Source: CAD feature listing. Evaluate the final solid. Frame: model axes, mm. A direction names the side the tool comes from. Round coordinates to 2 decimals unless told otherwise and drop trailing zeros. Loops run counter-clockwise (first coordinate to the right, second up) from the corner with the lowest first, then second, coordinate; pieces in that order, holes last. Notation, with made-up numbers: (-29, 32.25) - (-21, 32.25) arc R35 cw to (-21, 68.25) - close; hole circle Ø5 at (73, 66.25). An arc over 180 degrees is marked (long way). One line per question, with ' | ' between items. Start each with the question number.
1. Access query for faces 5 (the flat face through (-10, 7, 2)), 6 (the flat face through (-20, 70, 5)), 7 (the flat face through (13, 20, 5)). Directions: +Z, -Z, +X, -X, +Y, -Y. A direction counts if a zero-diameter tool reaches every point of the face in a straight line with its end or side. Return the directions, or none.
2. Cut plane D-D (z = 1). Return loops of the section in (x, y), then the cut area to 3 significant figures.
3. Cut plane C-C (z = -10). Return loops of the section in (x, y), then the cut area to 3 significant figures.
4. Pin query (flat end, axial travel): pin 1 (10 mm diameter, centred on y = 10.5, z = 4.5, fed in from +X); pin 2 (6.5 mm diameter, centred on x = 1, y = 43.5, fed in from +Z); pin 3 (3 mm diameter, centred on x = 14.5, y = 42, fed in from -Z); pin 4 (5 mm diameter, centred on x = 0, y = 47.5, fed in from -Z). Return the tip coordinate at first contact, or that it passes through.
5. Mould query, pull axis Y, two halves, no side actions, for faces 1 (the flat face through (0, 4, -13)), 2 (the flat face through (25, 47, 5)), 3 (the cylindrical face through (-2.379, 36.786, 6.549)), 4 (the cylindrical face through (0.14, 0.57, 9.4)). Classes: pulls with the +Y half, pulls with the -Y half, needs draft (parallel to the pull), parting line crosses it, or undercut.
6. Cut plane B-B (x = 0). Return loops of the section in (y, z) (3 decimals), then the cut area to 3 significant figures.
7. Cut plane A-A (y = 47.5). Return loops of the section in (x, z) (3 decimals).
8. Ray query, line 1 (Y direction, x = 0, z = 1.1); line 2 (Y direction, x = 0, z = 5.75) (3 decimals); line 3 (X direction, y = 1.1, z = -10). Return the intervals inside material, ascending.
```python
from build123d import *

# Parameters (mm, degrees)
SCHIZZO1_R                   = 4
ESTRUSIONE_ESTRUSIONE1_DEPTH = 10
SMUSSO1_SIZE                 = 10
SCHIZZO3_R                   = 10.975
TAGLIO_ESTRUSIONE1_DEPTH     = 7
SCHIZZO4_W                   = 20
SCHIZZO4_H                   = 4
ESTRUSIONE_ESTRUSIONE2_DEPTH = 20
RACCORDO1_R                  = 2
SCHIZZO5_R                   = 2.5
TAGLIO_ESTRUSIONE2_DEPTH     = 20
SCHIZZO6_R                   = 2.5
TAGLIO_ESTRUSIONE3_DEPTH     = 11


with BuildPart() as part:
    # Schizzo1 → Estrusione-Estrusione1 (new body)
    with BuildSketch(Plane.XY):
        Polygon((-25, 20), (-10, 20), (-10, 0), (10, 0), (10, 20), (25, 20), (25, 75), (-25, 75), align=None)
        with Locations((0, 47.5)):
            Circle(SCHIZZO1_R, mode=Mode.SUBTRACT)
    extrude(amount=ESTRUSIONE_ESTRUSIONE1_DEPTH)

    # Smusso1
    smusso1_edges = [part.edges().sort_by_distance(p)[0] for p in [
        (25, 20, 5),
        (-25, 20, 5),
        (-25, 75, 5),
        (25, 75, 5),
    ]]
    chamfer(smusso1_edges, length=SMUSSO1_SIZE)

    # Schizzo3 → Taglio-Estrusione1 (cut)
    with BuildSketch(Plane.XY.offset(10)):
        with Locations((0, 47.5)):
            Circle(SCHIZZO3_R)
    extrude(amount=-TAGLIO_ESTRUSIONE1_DEPTH, mode=Mode.SUBTRACT)

    # Schizzo4 → Estrusione-Estrusione2 (add)
    with BuildSketch(Plane(origin=(0, 0, 0), x_dir=(-1, 0, 0), z_dir=(0, 0, -1))):
        with Locations((0, 2)):
            Rectangle(SCHIZZO4_W, SCHIZZO4_H)
    extrude(amount=ESTRUSIONE_ESTRUSIONE2_DEPTH)

    # Raccordo1
    raccordo1_edges = [part.edges().sort_by_distance(p)[0] for p in [
        (10, 20, 5),
        (-10, 20, 5),
        (0, 0, 10),
        (0, 4, 0),
        (10, 2, -20),
        (-10, 2, -20),
    ]]
    fillet(raccordo1_edges, radius=RACCORDO1_R)

    # Schizzo5 → Taglio-Estrusione2 (cut)
    with BuildSketch(Plane(origin=(0, 4, 0), x_dir=(1, 0, 0), z_dir=(0, 1, 0))):
        with Locations((0, 10)):
            Circle(SCHIZZO5_R)
    extrude(amount=-TAGLIO_ESTRUSIONE2_DEPTH, mode=Mode.SUBTRACT)

    # Schizzo6 → Taglio-Estrusione3 (cut, through all)
    with BuildSketch(Plane(origin=(0, 0, 0), x_dir=(-1, 0, 0), z_dir=(0, 0, -1))):
        with Locations((0, 10)):
            Circle(SCHIZZO6_R)
    extrude(amount=-TAGLIO_ESTRUSIONE3_DEPTH, mode=Mode.SUBTRACT)


solid = part.part
```
Answers follow:
1) face 5: +Z, -Z, -X, -Y | face 6: +Z, -Z, -X, +Y | face 7: +Z, -Z, +X, -Y
2) outline: (-25, 30) - (-15, 20) - (-12, 20) arc R2 cw to (-10, 18) - (-10, 0) - (10, 0) - (10, 18) arc R2 cw to (12, 20) - (15, 20) - (25, 30) - (25, 65) - (15, 75) - (-15, 75) - (-25, 65) - close; hole circle Ø8 at (0, 47.5); hole circle Ø5 at (0, 10) | area: 2,880 mm2
3) outline: (-10, 0) - (-2.5, 0) - (-2.5, 4) - (-10, 4) - close; (2.5, 0) - (10, 0) - (10, 4) - (2.5, 4) - close | area: 60.0 mm2
4) pin 1: stops at x = 10 | pin 2: stops at z = 3 | pin 3: stops at z = 0 | pin 4: passes through
5) face 1: pulls with the +Y half | face 2: needs draft | face 3: undercut | face 4: pulls with the -Y half
6) outline: (0, -20) - (4, -20) - (4, -12.5) - (0, -12.5) - close; (0, -7.5) - (4, -7.5) - (4, -2) arc R2 cw to (6, 0) - (7.5, 0) - (7.5, 10) - (2, 10) arc R2 ccw to (0, 8) - close; (12.5, 0) - (43.5, 0) - (43.5, 3) - (36.525, 3) - (36.525, 10) - (12.5, 10) - close; (51.5, 0) - (75, 0) - (75, 10) - (58.475, 10) - (58.475, 3) - (51.5, 3) - close | area: 582 mm2
7) outline: (-25, 0) - (-4, 0) - (-4, 3) - (-10.975, 3) - (-10.975, 10) - (-25, 10) - close; (4, 0) - (25, 0) - (25, 10) - (10.975, 10) - (10.975, 3) - (4, 3) - close
8) line 1: y = 0 to 7.5, 12.5 to 43.5, 51.5 to 75 | line 2: y = 0 to 7.5, 12.5 to 36.525, 58.475 to 75 | line 3: x = -10 to -2.5, 2.5 to 10
